Build history of the part. All positions in model axes, mm. Round coordinates to 2 decimals unless told otherwise and drop trailing zeros. Order: outer loops, then holes, each group sorted by start corner. A loop starts at its lowest first (then second) coordinate and runs counter-clockwise, first axis right, second up. Notation, with made-up numbers: (33, 63) -> (89, 63) arc R30 ccw to (89, 90) -> close; hole circle Ø2 at (48, 35). An arc over 180 degrees is marked (long way). Write item = value, one per line.
from build123d import *

# Parameters (mm, degrees)
IZIM1_R                          = 3
Y_KSEKLIK_EKSTR_ZYON1_DEPTH      = 1
Y_KSEKLIK_EKSTR_ZYON1_DEPTH_BACK = 1
RADYUS1_R                        = 0.9
RADYUS2_R                        = 0.9
IZIM2_W                          = 0.358194198
IZIM2_H                          = 0.28655536
Y_KSEKLIK_EKSTR_ZYON2_DEPTH      = 0.7
Y_KSEKLIK_EKSTR_ZYON2_DEPTH_BACK = 2.7
IZIM3_R                          = 0.171322749
IZIM3_R_2                        = 0.177674655
Y_KSEKLIK_EKSTR_ZYON3_DEPTH      = 10
IZIM5_R                          = 0.171322749
Y_KSEKLIK_EKSTR_ZYON4_DEPTH      = 1.6
Y_KSEKLIK_EKSTR_ZYON4_DEPTH_BACK = 1.6
KES_EKSTR_ZYON1_DEPTH            = 1.6


with BuildPart() as part:
    # izim1 → Y_kseklik-Ekstr_zyon1 (new body, two sides)
    with BuildSketch(Plane(origin=(0, 0, 0), x_dir=(0, 0, -1), z_dir=(1, 0, 0))) as y_kseklik_ekstr_zyon1_sk:
        Circle(IZIM1_R)
    extrude(amount=Y_KSEKLIK_EKSTR_ZYON1_DEPTH)
    extrude(y_kseklik_ekstr_zyon1_sk.sketch, amount=-Y_KSEKLIK_EKSTR_ZYON1_DEPTH_BACK)

    # Radyus1
    radyus1_edges = [part.edges().sort_by_distance(p)[0] for p in [
        (-1, 0, 3),
    ]]
    fillet(radyus1_edges, radius=RADYUS1_R)

    # Radyus2
    radyus2_edges = [part.edges().sort_by_distance(p)[0] for p in [
        (1, 0, 3),
    ]]
    fillet(radyus2_edges, radius=RADYUS2_R)

    # izim2 → Y_kseklik-Ekstr_zyon2 (add, two sides)
    with BuildSketch(Plane(origin=(1, 0, 0), x_dir=(0, 0, -1), z_dir=(1, 0, 0))) as y_kseklik_ekstr_zyon2_sk:
        Rectangle(IZIM2_W, IZIM2_H)
    extrude(amount=Y_KSEKLIK_EKSTR_ZYON2_DEPTH)
    extrude(y_kseklik_ekstr_zyon2_sk.sketch, amount=-Y_KSEKLIK_EKSTR_ZYON2_DEPTH_BACK)

    # izim3 → Y_kseklik-Ekstr_zyon3 (add)
    with BuildSketch(Plane(origin=(0, 0, 0), x_dir=(1, 0, 0), z_dir=(0, 1, 0))):
        with Locations((-1.529245006, 0)):
            Circle(IZIM3_R)
        with Locations((1.522325345, 0)):
            Circle(IZIM3_R_2)
    extrude(amount=Y_KSEKLIK_EKSTR_ZYON3_DEPTH)

    # izim5 → Y_kseklik-Ekstr_zyon4 (add, two sides)
    with BuildSketch(Plane(origin=(0, 0, 0), x_dir=(0, 0, -1), z_dir=(1, 0, 0))) as y_kseklik_ekstr_zyon4_sk:
        with Locations((0, 6.037482004)):
            Circle(IZIM5_R)
    extrude(amount=Y_KSEKLIK_EKSTR_ZYON4_DEPTH)
    extrude(y_kseklik_ekstr_zyon4_sk.sketch, amount=-Y_KSEKLIK_EKSTR_ZYON4_DEPTH_BACK)

    # izim6 → D_nd_r-_nce1 (revolve)
    with BuildSketch(Plane(origin=(0, 0, 0), x_dir=(0, 0, -1), z_dir=(1, 0, 0))):
        Polygon((-0.156029533, 6.037482004), (-3.82275516, 10), (-3.896152209, 9.932081863), (-0.229426581, 5.969563868), align=None)
    revolve(axis=Axis((0, 6.037482004, 0.156029533), (0, 0.733970484, 0.679181366)))

    # izim7 → Kes-Ekstr_zyon1 (cut)
    with BuildSketch(Plane(origin=(0, 10, 0), x_dir=(1, 0, 0), z_dir=(0, 1, 0))):
        Polygon((-0.387982537, -3.298594138), (-0.387982537, -3.511184794), (-0.387982537, -4.384499274), (0.201510503, -4.384499274), (0.201510503, -3.298594138), align=None)
    extrude(amount=KES_EKSTR_ZYON1_DEPTH, mode=Mode.SUBTRACT)


solid = part.part
Q1. Cut at A-A, the plane x = -1.15. List the corners of the cut face in (y, z).
Check values:
outline = (-0.14, -0.18) -> (0.14, -0.18) -> (0.14, 0.18) -> (-0.14, 0.18) -> close; circle Ø0.34 at (6.04, 0)
Q2. Probe probe 1 along X at (y, z) = (2, 0.5); probe 2 along Y at (x, z) = (0.65, 0); probe 3 along Y at (x, z) = (0.2, 0). List the from-to ranges inside material, lowest first.
Check values:
probe_1 = -1 to 1
probe_2 = -2.81 to 2.81, 5.87 to 6.21
probe_3 = -2.99 to 2.99, 5.87 to 6.21
Q3. Flat gauge pins, fed straight in: pin 1 (1 mm diameter, centred on y = 1, z = 3, fed in from -X); pin 2 (1 mm diameter, centred on x = 0.5, y = 4.5, fed in from -Z); pin 3 (1.5 mm diameter, centred on x = -1, z = 2, fed in from +Y). Where does each tip first touch, or does it go through?
Check values:
pin_1 = -0.8
pin_2 = through
pin_3 = 2.52
Q4. Cut at B-B, the plane y = 5. List the corners of the cut face in (x, z).
Check values:
outline = circle Ø0.34 at (-1.53, 0); circle Ø0.36 at (1.52, 0)
Q5. Cut at C-C, the plane y = 9. Give the number of separate pieces and of enclosed holes in the cut face, and give its area (3 significant figures).
Check values:
separate_pieces = 3
enclosed_holes = 0
area = 0.234 mm²
